```python
from build123d import *

# Parameters (mm, degrees)
BOSS_EXTRUDE1_DEPTH = 60
SKETCH3_W           = 400
SKETCH3_H           = 300
CUT_EXTRUDE1_DEPTH  = 41
BOSS_EXTRUDE2_DEPTH = 350
BOSS_EXTRUDE3_DEPTH = 350
FILLET1_R           = 50
FILLET2_R           = 50
SKETCH6_W           = 253
SKETCH6_H           = 320
SKETCH6_W_2         = 384.289648178
SKETCH6_H_2         = 327.7
BOSS_EXTRUDE4_DEPTH = 31
CHAMFER5_SIZE       = 10
FILLET3_R           = 5


with BuildPart() as part:
    # Sketch1 → Boss-Extrude1 (new body)
    with BuildSketch(Plane(origin=(0, 0, 0), x_dir=(1, 0, 0), z_dir=(0, 1, 0))):
        Polygon((818, 792.7), (0, 792.7), (0, 0), (482.77197137, 0), (818, 309.005759394), align=None)
    extrude(amount=BOSS_EXTRUDE1_DEPTH)

    # Sketch3 → Cut-Extrude1 (cut)
    with BuildSketch(Plane(origin=(0, 60, 0), x_dir=(1, 0, 0), z_dir=(0, 1, 0))):
        with Locations((250, 592.7)):
            Rectangle(SKETCH3_W, SKETCH3_H)
        Polygon((168.605055776, 392.7), (500, 392.7), (500, 678.249343647), (500, 742.7), (768, 742.7), (768, 329.953464166), (464.289648178, 50), (50, 50), (50, 392.7), align=None)
    extrude(amount=-CUT_EXTRUDE1_DEPTH, mode=Mode.SUBTRACT)

    # Sketch4 → Boss-Extrude2 (add)
    with BuildSketch(Plane(origin=(0, 19, 0), x_dir=(1, 0, 0), z_dir=(0, 1, 0))):
        Polygon((464.289648178, 50), (464.289648178, 392.7), (449.289648178, 392.7), (449.289648178, 65), (65, 65), (65, 392.7), (50, 392.7), (50, 50), align=None)
    extrude(amount=BOSS_EXTRUDE2_DEPTH)

    # Sketch5 → Boss-Extrude3 (add)
    with BuildSketch(Plane(origin=(0, 19, 0), x_dir=(1, 0, 0), z_dir=(0, 1, 0))):
        Polygon((768, 392.7), (768, 742.7), (500, 742.7), (500, 727.7), (753, 727.7), (753, 407.7), (500, 407.7), (449.289648178, 407.7), (449.289648178, 392.7), align=None)
    extrude(amount=BOSS_EXTRUDE3_DEPTH)

    # Fillet1
    fillet1_edges = [part.edges().sort_by_distance(p)[0] for p in [
        (57.5, 369, -392.7),
        (500, 369, -735.2),
    ]]
    fillet(fillet1_edges, radius=FILLET1_R)

    # Fillet2
    fillet2_edges = [part.edges().sort_by_distance(p)[0] for p in [
        (0, 30, 0),
        (0, 30, -792.7),
        (818, 30, -792.7),
        (818, 30, -309.005759394),
        (482.77197137, 30, 0),
    ]]
    fillet(fillet2_edges, radius=FILLET2_R)

    # Sketch6 → Boss-Extrude4 (add)
    with BuildSketch(Plane(origin=(0, 19, 0), x_dir=(1, 0, 0), z_dir=(0, 1, 0))):
        Polygon((768, 392.7), (464.289648178, 392.7), (464.289648178, 50), (768, 329.953464166), align=None)
        with Locations((626.5, 567.7)):
            Rectangle(SKETCH6_W, SKETCH6_H)
        with Locations((257.144824089, 228.85)):
            Rectangle(SKETCH6_W_2, SKETCH6_H_2)
    extrude(amount=BOSS_EXTRUDE4_DEPTH)

    # Chamfer5
    chamfer5_edges = [part.edges().sort_by_distance(p)[0] for p in [
        (753, 50, -567.7),
        (626.5, 50, -727.7),
        (500, 50, -567.7),
        (626.5, 50, -407.7),
        (449.289648178, 50, -228.85),
        (257.144824089, 50, -392.7),
        (65, 50, -228.85),
        (257.144824089, 50, -65),
    ]]
    chamfer(chamfer5_edges, length=CHAMFER5_SIZE - 0.0001)  # a hair under: the kernel refuses the full size

    # Fillet3
    fillet3_edges = [part.edges().sort_by_distance(p)[0] for p in [
        (50, 214.5, -50),
        (464.289648178, 214.5, -50),
        (768, 214.5, -392.7),
        (768, 214.5, -742.7),
    ]]
    fillet(fillet3_edges, radius=FILLET3_R)


solid = part.part
```
Can you work these out from the model? Positions are in its coordinate system, mm. A direction names the side the tool comes from. Give positions to 0.01 mm unless a question says otherwise; leave off trailing zeros. Order: outer loops, then holes, each group sorted by start corner. A loop starts at its lowest first (then second) coordinate and runs counter-clockwise, first axis right, second up. Notation, with made-up numbers: (-27.75, 85) - (-15.75, 85) arc R26 cw to (-15.75, 114) - close; hole circle Ø10 at (-23, -6.5). An arc over 180 degrees is marked (long way). Use a Markdown table: item, result. Add a question column.
Q1. On a 3-axis mill with a long thin cutter (end or side, diameter ignored), from which of +Z, -Z, +X, -X, +Y, -Y can I reach the whole of each face in a straight line? I mean faces 1 (the flat face through (753, 212, -570)), 2 (the flat face through (449.29, 212, -239)), 3 (the flat face through (50, 212, -226)), 4 (the flat face through (255, 50, -231)). Say none if no direction works.
Q2. If we mould it in two halves opening along X, with no side actions, what happens to faces 5 (the cylindrical face through (514.258, 353.964, -735.095)), 6 (the flat face through (247, 40, -442.7)), 7 (the flat face through (403, 0, -402)), 8 (the flat face through (647.38, 29.58, -151.73))? For each: released by +X, released by -X, zero draft, split by the parting line, or undercut.
Q3. I'm going to push flat-ended pins straight in: pin 1 (1 mm diameter, centred on x = 299, z = -396.5, fed in from +Y); pin 2 (10 mm diameter, centred on x = 401.5, y = 192, fed in from -Z); pin 3 (4 mm diameter, centred on y = 76, z = -411.5, fed in from +X). Where does each tip first touch, or does it pass through?
Q4. Please list where these lines run through material, in increasing order: line 1 along X through (y, z) = (228.5, -352); line 2 along X through (y, z) = (25, -475.5); line 3 along Y through (x, z) = (381, -662.5).
Q5. If we section it at A-A on y = 251: Write out the boundary of the cut face in (x, z), plus the area to 3 significant figures.
Q6. If we section it at D-D on y = 345: Write out the boundary of the cut face in (x, z).
Answers follow:
| question | item | result |
|---|---|---|
| 1 | face 1 | -X, +Y |
| 1 | face 2 | -Z, +Y |
| 1 | face 3 | +Z, -Z, -X, +Y |
| 1 | face 4 | +Y |
| 2 | face 5 | released by -X |
| 2 | face 6 | undercut |
| 2 | face 7 | zero draft |
| 2 | face 8 | released by +X |
| 3 | pin 1 | stops at y = 60 |
| 3 | pin 2 | stops at z = -65 |
| 3 | pin 3 | stops at x = 768 |
| 4 | line 1 | x = 50 to 65, 449.29 to 464.29 |
| 4 | line 2 | x = 0 to 50, 450 to 818 |
| 4 | line 3 | y = 0 to 19 |
| 5 | outline | (50, -392.7) - (65, -392.7) - (65, -65) - (449.29, -65) - (449.29, -407.7) - (753, -407.7) - (753, -727.7) - (500, -727.7) - (500, -742.7) - (763, -742.7) arc R5 ccw to (768, -737.7) - (768, -397.7) arc R5 ccw to (763, -392.7) - (464.29, -392.7) - (464.29, -55) arc R5 ccw to (459.29, -50) - (55, -50) arc R5 ccw to (50, -55) - close |
| 5 | area | 29,600 mm^2 |
| 6 | outline | (50, -385.41) - (65, -385.41) - (65, -65) - (449.29, -65) - (449.29, -407.7) - (753, -407.7) - (753, -727.7) - (507.29, -727.7) - (507.29, -742.7) - (763, -742.7) arc R5 ccw to (768, -737.7) - (768, -397.7) arc R5 ccw to (763, -392.7) - (464.29, -392.7) - (464.29, -55) arc R5 ccw to (459.29, -50) - (55, -50) arc R5 ccw to (50, -55) - close |
